Verification items for the finished model (mm, model axes). A direction names the side the tool comes from. Round coordinates to 2 decimals unless told otherwise and drop trailing zeros. Write each loop counter-clockwise with the first axis right and the second up, starting at its lowest first coordinate (ties: lowest second). Pieces come first, ordered by that corner, then holes. Notation, with made-up numbers: (71.5, 19) - (120.5, 19) arc R10 ccw to (120.5, 27) - close; hole circle Ø1 at (-6.75, 48.25). An arc over 180 degrees is marked (long way). Write each question's results on one line, items separated by ' | '.
```python
from build123d import *

# Parameters (mm, degrees)
SKETCH1_W           = 309.5625
SKETCH1_H           = 231.775
SKETCH1_W_2         = 265.1125
SKETCH1_H_2         = 187.325
SKETCH1_W_3         = 227.0125
SKETCH1_H_3         = 150.8125
BOSS_EXTRUDE1_DEPTH = 9.525
SKETCH1_3_W         = 265.1125
SKETCH1_3_H         = 187.325
SKETCH1_3_W_2       = 227.0125
SKETCH1_3_H_2       = 150.8125
BOSS_EXTRUDE2_DEPTH = 6.35
FILLET1_R           = 12.7
CUT_EXTRUDE1_START  = 9.525
SKETCH1_4_W         = 265.1125
SKETCH1_4_H         = 187.325
SKETCH1_4_W_2       = 227.0125
SKETCH1_4_H_2       = 150.8125
CUT_EXTRUDE1_DEPTH  = 6.35
FILLET2_R           = 6.35
FILLET3_R           = 12.7
FILLET4_R           = 9.525


with BuildPart() as part:
    # Sketch1 → Boss-Extrude1 (new body)
    # profile 1 of 2: a face of its own
    with BuildSketch(Plane.XY):
        Rectangle(SKETCH1_W, SKETCH1_H)
        Rectangle(SKETCH1_W_2, SKETCH1_H_2, mode=Mode.SUBTRACT)
    # profile 2 of 2: a face of its own
    with BuildSketch(Plane.XY):
        Rectangle(SKETCH1_W_2, SKETCH1_H_2)
        Rectangle(SKETCH1_W_3, SKETCH1_H_3, mode=Mode.SUBTRACT)
    extrude(amount=BOSS_EXTRUDE1_DEPTH)

    # Sketch1<3> → Boss-Extrude2 (add)
    with BuildSketch(Plane.XY):
        Rectangle(SKETCH1_3_W, SKETCH1_3_H)
        Rectangle(SKETCH1_3_W_2, SKETCH1_3_H_2, mode=Mode.SUBTRACT)
    extrude(amount=-BOSS_EXTRUDE2_DEPTH)

    # Fillet1
    fillet1_edges = [part.edges().sort_by_distance(p)[0] for p in [
        (-154.78125, -115.8875, 4.7625),
        (-154.78125, 115.8875, 4.7625),
        (154.78125, 115.8875, 4.7625),
        (154.78125, -115.8875, 4.7625),
        (132.55625, -93.6625, -3.175),
        (-132.55625, -93.6625, -3.175),
        (-132.55625, 93.6625, -3.175),
        (132.55625, 93.6625, -3.175),
    ]]
    fillet(fillet1_edges, radius=FILLET1_R)

    # Sketch1<4> → Cut-Extrude1 (cut)
    with BuildSketch(Plane.XY.offset(CUT_EXTRUDE1_START)):
        Rectangle(SKETCH1_4_W, SKETCH1_4_H)
        Rectangle(SKETCH1_4_W_2, SKETCH1_4_H_2, mode=Mode.SUBTRACT)
    extrude(amount=-CUT_EXTRUDE1_DEPTH, mode=Mode.SUBTRACT)

    # Fillet2
    fillet2_edges = [part.edges().sort_by_distance(p)[0] for p in [
        (-113.50625, 75.40625, -1.5875),
        (113.50625, 75.40625, -1.5875),
        (-113.50625, -75.40625, -1.5875),
        (113.50625, -75.40625, -1.5875),
    ]]
    fillet(fillet2_edges, radius=FILLET2_R)

    # Fillet3
    fillet3_edges = [part.edges().sort_by_distance(p)[0] for p in [
        (-132.55625, -93.6625, 6.35),
        (-132.55625, 93.6625, 6.35),
        (132.55625, 93.6625, 6.35),
        (132.55625, -93.6625, 6.35),
    ]]
    fillet(fillet3_edges, radius=FILLET3_R)

    # Fillet4
    fillet4_edges = [part.edges().sort_by_distance(p)[0] for p in [
        (-151.061506121, -112.167756121, 9.525),
        (0, -115.8875, 9.525),
        (151.061506121, -112.167756121, 9.525),
        (154.78125, 0, 9.525),
        (151.061506121, 112.167756121, 9.525),
        (0, 115.8875, 9.525),
        (-151.061506121, 112.167756121, 9.525),
        (-154.78125, 0, 9.525),
    ]]
    fillet(fillet4_edges, radius=FILLET4_R - 0.0001)  # a hair under: the kernel refuses the full size


solid = part.part
```
(1) Set-up check for faces 1 (the flat face through (132.556, -1, -3)), 2 (the cylindrical face through (-111.597, 73.595, -1.654)), 3 (the flat face through (-2, 93.662, 6)), 4 (the cylindrical face through (128.935, -89.843, -3.219)): record each of +Z, -Z, +X, -X, +Y, -Y from which the full face is reachable in a straight line by a thin tool's end or side.
Answer:
face 1: -Z, +X, +Y, -Y | face 2: +Z, -Z | face 3: +Z | face 4: -Z, +X, -Y
(2) Go/stop test with flat-tipped pins: pin 1 Ø2 at (y, z) = (73, 3.5) entering from -X; pin 2 Ø1.9 at (x, z) = (28, -2.5) entering from +Y; pin 3 Ø1.5 at (x, z) = (-100, 2.5) entering from +Y. Record where each tip stops, or that it passes through.
Answer:
pin 1: x = -154.45 | pin 2: y = 93.66 | pin 3: y = 115.73
(3) Thickness scan on L1, parallel to X at y = 53.5, z = -2; L2, parallel to X at y = 40, z = 0.75; L3, parallel to Y at x = 58.5, z = -4. Record the ranges inside material, lowest first.
Answer:
L1: -132.56 to -113.51, 113.51 to 132.56 | L2: -154.75 to -113.51, 113.51 to 154.75 | L3: -93.66 to -75.41, 75.41 to 93.66
(4) Mould release check, pull along Y, two halves, no side actions. Record for faces 5 (the flat face through (-2, 93.662, -3)), 6 (the flat face through (-2, -93.662, 6)), 7 (the cylindrical face through (151.917, -1.445, 6.809)), 8 (the flat face through (132.556, -1, 6)): released by +Y, released by -Y, zero draft, split by the parting line, or undercut.
Answer:
face 5: released by +Y | face 6: undercut | face 7: zero draft | face 8: undercut
(5) Section check B-B (z = -3.5). Record the cut outline in (x, y).
Answer:
outline: (-132.56, -80.96) arc R12.7 ccw to (-119.86, -93.66) - (119.86, -93.66) arc R12.7 ccw to (132.56, -80.96) - (132.56, 80.96) arc R12.7 ccw to (119.86, 93.66) - (-119.86, 93.66) arc R12.7 ccw to (-132.56, 80.96) - close; hole (-113.51, -69.06) arc R6.35 ccw to (-107.16, -75.41) - (107.16, -75.41) arc R6.35 ccw to (113.51, -69.06) - (113.51, 69.06) arc R6.35 ccw to (107.16, 75.41) - (-107.16, 75.41) arc R6.35 ccw to (-113.51, 69.06) - close
